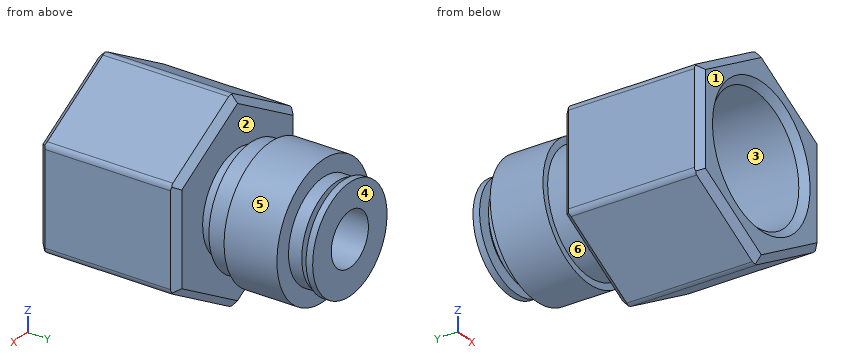
from build123d import *

# Parameters (mm, degrees)
EXTRUDE_1_DEPTH          = 21
SKETCH_2_R               = 7.5
EXTRUDE_2_DEPTH          = 2
SKETCH_3_R               = 9
EXTRUDE_3_DEPTH          = 3
SKETCH_4_R               = 10
EXTRUDE_4_DEPTH          = 8
SKETCH_5_R               = 7.5
EXTRUDE_5_DEPTH          = 2
CUT_EXTRUDE_1_DEPTH      = 42.106568818
CUT_EXTRUDE_1_DEPTH_BACK = 42.106568818
SKETCH_7_R               = 4
HOLE_WIZARD_G1_21_D      = 19
HOLE_WIZARD_G1_21_DEPTH  = 18
HOLE_WIZARD_G1_21_TIP    = 5.708175881
CHAMFER_1_SIZE           = 1
FILLET_1_R               = 1


with BuildPart() as part:
    # Эскиз1 → Бобышка-Вытянуть1 (new body)
    with BuildSketch(Plane(origin=(0, 0, 0), x_dir=(1, 0, 0), z_dir=(0, 1, 0))):
        Polygon((0, 15), (-12.990381057, 7.5), (-12.990381057, -7.5), (0, -15), (12.990381057, -7.5), (12.990381057, 7.5), align=None)
    extrude(amount=EXTRUDE_1_DEPTH)

    # Эскиз2 → Бобышка-Вытянуть2 (add)
    with BuildSketch(Plane(origin=(0, 21, 0), x_dir=(1, 0, 0), z_dir=(0, 1, 0))):
        with Locations(Location((0, 0, 0), (0, 0, 270))):
            Circle(SKETCH_2_R)
    extrude(amount=EXTRUDE_2_DEPTH)

    # Эскиз3 → Бобышка-Вытянуть3 (add)
    with BuildSketch(Plane(origin=(0, 23, 0), x_dir=(1, 0, 0), z_dir=(0, 1, 0))):
        with Locations(Location((0, 0, 0), (0, 0, 270))):
            Circle(SKETCH_3_R)
    extrude(amount=EXTRUDE_3_DEPTH)

    # Эскиз4 → Бобышка-Вытянуть4 (add)
    with BuildSketch(Plane(origin=(0, 26, 0), x_dir=(1, 0, 0), z_dir=(0, 1, 0))):
        with Locations(Location((0, 0, 0), (0, 0, 270))):
            Circle(SKETCH_4_R)
    extrude(amount=EXTRUDE_4_DEPTH)

    # Эскиз5 → Бобышка-Вытянуть5 (add)
    with BuildSketch(Plane(origin=(0, 34, 0), x_dir=(1, 0, 0), z_dir=(0, 1, 0))):
        with Locations(Location((0, 0, 0), (0, 0, 270))):
            Circle(SKETCH_5_R)
    extrude(amount=EXTRUDE_5_DEPTH)

    # Эскиз6 → Повернуть1 (revolve)
    with BuildSketch(Plane.XY, mode=Mode.PRIVATE) as revolve_1_sk:
        Polygon((-8, 37), (-6, 37), (-6, 36), (-4, 36), (-4, 38), (-8, 38), align=None)
    revolve(revolve_1_sk.sketch.rotate(Axis((0, 36, 0), (0, 1, 0)), 270), axis=Axis((0, 36, 0), (0, 1, 0)))

    # Эскиз7 → Вырез-Вытянуть1 (cut, two sides: drawn at the far end of the back side and taken through both)
    with BuildSketch(Plane(origin=(0, 36, 0), x_dir=(1, 0, 0), z_dir=(0, 1, 0)).offset(-CUT_EXTRUDE_1_DEPTH_BACK)):
        with Locations(Location((0, 0, 0), (0, 0, 90))):
            Circle(SKETCH_7_R)
    extrude(amount=CUT_EXTRUDE_1_DEPTH + CUT_EXTRUDE_1_DEPTH_BACK, mode=Mode.SUBTRACT)

    # Отверстие обработанное метчиком G1/21
    with Locations(Plane(origin=(0, 0, 0), x_dir=(-1, 0, 0), z_dir=(0, -1, 0))):
        with Locations((0, 0)):
            Hole(HOLE_WIZARD_G1_21_D / 2, depth=HOLE_WIZARD_G1_21_DEPTH)
            with Locations((0, 0, -(HOLE_WIZARD_G1_21_DEPTH + HOLE_WIZARD_G1_21_TIP / 2))):  # 118° drill point
                Cone(0, HOLE_WIZARD_G1_21_D / 2, HOLE_WIZARD_G1_21_TIP, mode=Mode.SUBTRACT)

    # Фаска1
    chamfer_1_edges = [part.edges().sort_by_distance(p)[0] for p in [
        (-12.990381057, 21, 0),
        (-6.495190528, 21, 11.25),
        (6.495190528, 21, 11.25),
        (12.990381057, 21, 0),
        (6.495190528, 21, -11.25),
        (-9.5, 0, 0),
        (12.990381057, 0, 0),
        (6.495190528, 0, 11.25),
        (-6.495190528, 0, 11.25),
        (-6.495190528, 21, -11.25),
        (-12.990381057, 0, 0),
        (-6.495190528, 0, -11.25),
        (6.495190528, 0, -11.25),
    ]]
    chamfer(chamfer_1_edges, length=CHAMFER_1_SIZE)

    # Скругление1
    fillet_1_edges = [part.edges().sort_by_distance(p)[0] for p in [
        (12.990381057, 10.5, -7.5),
        (12.990381057, 10.5, 7.5),
        (0, 10.5, 15),
        (-12.990381057, 10.5, 7.5),
        (-12.990381057, 10.5, -7.5),
        (0, 10.5, -15),
    ]]
    fillet(fillet_1_edges, radius=FILLET_1_R)


solid = part.part
The listing builds one solid part. Answer for the finished solid, in the listing's coordinates (mm). Face numbers are marked on the shaded views. A direction names the side the tool comes from. Give positions to 0.01 mm unless a question says otherwise; leave off trailing zeros. Order: outer loops, then holes, each group sorted by start corner. A loop starts at its lowest first (then second) coordinate and runs counter-clockwise, first axis right, second up. Notation, with made-up numbers: (81.25, 25.25) - (95.25, 25.25) arc R28 cw to (95.25, 61.25) - close; hole circle Ø8 at (60, 65). An arc over 180 degrees is marked (long way). Answer as CSV lines item,"result".
Q1. A cutting plane is placed at C-C, the plane y = 31.5. Determine the outline of the cut face in (x, z).
Answer key:
outline,"circle Ø20 at (0, 0); hole circle Ø8 at (0, 0)"
Q2. Straight lines are drawn through the part: L1, parallel to Z at x = 0, y = 10.5; L2, parallel to Y at x = -3.5, z = -6.75; L3, parallel to X at y = 14, z = 0. For each, find the intervals that lie inside material, in ascending order.
Answer key:
L1,"z = -14.85 to -9.5, 9.5 to 14.85"
L2,"y = 19.14 to 21, 23 to 34, 37 to 38"
L3,"x = -12.99 to -9.5, 9.5 to 12.99"
Q3. A cutting plane is placed at B-B, the plane y = 25.5. Determine the outline of the cut face in (x, z).
Answer key:
outline,"circle Ø18 at (0, 0); hole circle Ø8 at (0, 0)"
Q4. Which of the six approach directions +Z, -Z, +X, -X, +Y, -Y give full straight-line access (tool end or side, diameter ignored) to the marked faces 4, 5 and 6?
Answer key:
face 4,"+Z, -Z, +X, -X, +Y"
face 5,"+Y"
face 6,"none"
Q5. Determine the mould class of the marked faces 1, 2 and 3 for opening direction Y: pulls with the +Y half, pulls with the -Y half, needs draft (parallel to the pull), parting line crosses it, or undercut.
Answer key:
face 1,"pulls with the -Y half"
face 2,"undercut"
face 3,"needs draft"
Q6. Each of these flat-tipped pins is pushed along its axis until it touches: pin 1 Ø10 at (x, z) = (-1, 0.5) entering from -Y; pin 2 Ø10 at (x, z) = (-8.5, 10) entering from +Y; pin 3 Ø9 at (x, z) = (0, 3) entering from -Y; pin 4 Ø5 at (x, z) = (0, 0) entering from -Y. Where does it stop, or does it pass through?
Answer key:
pin 1,"stops at y = 20.03"
pin 2,"stops at y = 34"
pin 3,"stops at y = 19.2"
pin 4,"passes through"
Q7. A cutting plane is placed at A-A, the plane y = 9.5. Determine the outline of the cut face in (x, z).
Answer key:
outline,"(-12.99, -6.92) arc R1 ccw to (-12.49, -7.79) - (-0.5, -14.71) arc R1 ccw to (0.5, -14.71) - (12.49, -7.79) arc R1 ccw to (12.99, -6.92) - (12.99, 6.92) arc R1 ccw to (12.49, 7.79) - (0.5, 14.71) arc R1 ccw to (-0.5, 14.71) - (-12.49, 7.79) arc R1 ccw to (-12.99, 6.92) - close; hole circle Ø19 at (0, 0)"
